Model file for the job. Use its own axes, mm. A direction names the side the tool comes from. Give positions to 0.01 mm unless a question says otherwise; leave off trailing zeros. Loops run counter-clockwise (first coordinate to the right, second up) from the corner with the lowest first, then second, coordinate; pieces in that order, holes last. Notation, with made-up numbers: (-20.75, 73.25) -> (2.25, 73.25) arc R38 cw to (2.25, 111.25) -> close; hole circle Ø3 at (73.5, 41). An arc over 180 degrees is marked (long way). Use CSV: the item, a comma, the result in double quotes. Start each with the question number.
(1) Drill centre lines: probe 1 along X at (y, z) = (70, 9); probe 2 along Y at (x, z) = (19, 7.5); probe 3 along Z at (x, y) = (13.5, 69.25). Where is each one in solid material? Low to high.
(2) Flat gauge pin, fed straight in: pin 1 (1 mm diameter, centred on x = 35, y = 84, fed in from +Z). Where does the tip first touch, or does it go through?
(3) Pull direction X, two halves, no side cores. Call faces 1 (the flat face through (-1.305, 76, 5)), 2 (the flat face through (75.09, 76, 7)), 3 (the flat face through (39, 89.506, 5)): pulls with the +X half, pulls with the -X half, needs draft (parallel to the pull), parting line crosses it, or undercut.
(4) Cut at C-C on y = 72.75. Write the cut outline in (x, z).
(5) Cut at A-A on z = 8. Write the cut outline in (x, y).
(6) Cut at B-B on x = 14.5. Write the cut outline in (y, z), then the cut area to 3 significant figures.
(7) 3-axis set-ups, long thin cutter, end or side, ignore diameter. For faces 4 (the flat face through (38, 76, 0)), 5 (the flat face through (40, 84.705, 7)): which of +Z, -Z, +X, -X, +Y, -Y reach the whole face in a straight line?
Autodesk Fusion 360 part; units mm, degrees
box "BoxPrimitive2" add length 27 width 80 height 10 placed x (0, 1, 0) y (-1, 0, 0) z (0, 0, 1) at (78.6953, 62.5055, 0)
sketch "Sketch3" plane through (0, 0, 10) normal (0, 0, 1) x (-1, 0, 0)
  line L0 (-78.6953, -89.5055) -> (1.3047, -89.5055)
  line L1 (1.3047, -89.5055) -> (1.3047, -62.5055)
  line L2 (1.3047, -62.5055) -> (-78.6953, -62.5055)
  line L3 (-78.6953, -62.5055) -> (-78.6953, -89.5055)
  line L4 (-5.0904, -84.7047) -> (-75.0904, -84.7047)
  line L5 (-75.0904, -84.7047) -> (-75.0904, -67.7047)
  line L6 (-75.0904, -67.7047) -> (-5.0904, -67.7047)
  line L7 (-5.0904, -67.7047) -> (-5.0904, -84.7047)
  dimension "d16" = 70
  dimension "d17" = 17
extrude "Extrude1" cut sketch "Sketch3" against normal blind 6 contours L4 L5 L6 L7
Check result:
1,probe 1,"-1.3 to 5.09, 75.09 to 78.7"
1,probe 2,"62.51 to 67.7, 84.7 to 89.51"
1,probe 3,"0 to 4"
2,pin 1,"z = 4"
3,face 1,"pulls with the -X half"
3,face 2,"undercut"
3,face 3,"needs draft"
4,outline,"(-1.3, 0) -> (78.7, 0) -> (78.7, 10) -> (75.09, 10) -> (75.09, 4) -> (5.09, 4) -> (5.09, 10) -> (-1.3, 10) -> close"
5,outline,"(-1.3, 62.51) -> (78.7, 62.51) -> (78.7, 89.51) -> (-1.3, 89.51) -> close; hole (5.09, 67.7) -> (75.09, 67.7) -> (75.09, 84.7) -> (5.09, 84.7) -> close"
6,outline,"(62.51, 0) -> (89.51, 0) -> (89.51, 10) -> (84.7, 10) -> (84.7, 4) -> (67.7, 4) -> (67.7, 10) -> (62.51, 10) -> close"
6,area,"168 mm²"
7,face 4,"-Z, +X, -X, +Y, -Y"
7,face 5,"+Z"
